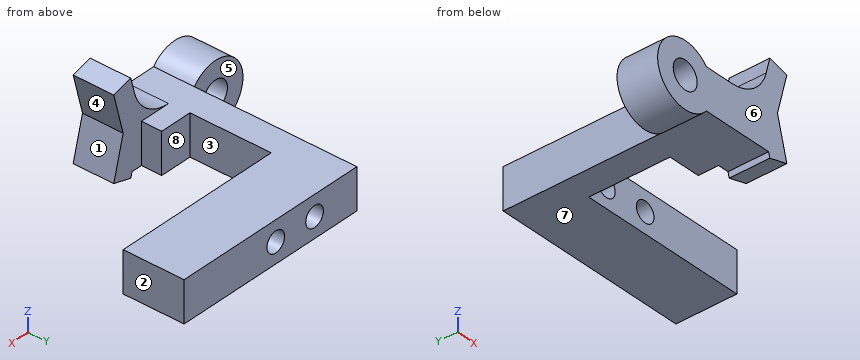
```python
from build123d import *

# Parameters (mm, degrees)
BOSS_EXTRUDE1_DEPTH = 5
BOSS_EXTRUDE2_DEPTH = 10
FILLET1_R           = 10
SKETCH3_W           = 8
SKETCH3_H           = 20
CUT_EXTRUDE1_DEPTH  = 74.171272574
SKETCH4_R           = 2.5
CUT_EXTRUDE2_DEPTH  = 63.379394923
SKETCH5_R           = 3.4
BOSS_EXTRUDE4_DEPTH = 10


with BuildPart() as part:
    # Sketch1 → Boss-Extrude1 (new, symmetric)
    with BuildSketch(Plane.XY):
        Polygon((49, 0), (0, 0), (0, -50), (15, -50), (15, -15), (49, -15), align=None)
    extrude(amount=BOSS_EXTRUDE1_DEPTH, both=True)

    # Sketch2 → Boss-Extrude2 (add)
    with BuildSketch(Plane.XZ.offset(50)):
        Polygon((22.832157544, -5), (18, -6.284621916), (15, 5), (18, 16.284621916), (22.832157544, 15), (20.173672375, 5), align=None)
        Polygon((15, -5), (17.658485169, -5), (15, 5), align=None)
        Polygon((18, 16.284621916), (15, 5), (20.173672375, 5), (22.832157544, 15), align=None)
    extrude(amount=-BOSS_EXTRUDE2_DEPTH)

    # Fillet1
    fillet1_edges = [part.edges().sort_by_distance(p)[0] for p in [
        (15, -45, 5),
    ]]
    fillet(fillet1_edges, radius=FILLET1_R)

    # Sketch3 → Cut-Extrude1 (cut, through all)
    with BuildSketch(Plane(origin=(0, 0, -5), x_dir=(-1, 0, 0), z_dir=(0, 0, -1))):
        with Locations((-11, -25)):
            Rectangle(SKETCH3_W, SKETCH3_H)
    extrude(amount=-CUT_EXTRUDE1_DEPTH, mode=Mode.SUBTRACT)

    # Sketch4 → Cut-Extrude2 (cut, through all)
    with BuildSketch(Plane.XZ.offset(15)):
        with Locations(Location((23, 0, 0), (0, 0, 270))):
            Circle(SKETCH4_R)
        with Locations(Location((12, 0, 0), (0, 0, 270))):
            Circle(SKETCH4_R)
    extrude(amount=-CUT_EXTRUDE2_DEPTH, mode=Mode.SUBTRACT)

    # Sketch5 → Boss-Extrude4 (add)
    with BuildSketch(Plane.XZ.offset(50)):
        with BuildLine():
            Line((0, 5), (0, -5))
            ThreePointArc((0, -5), (-13.810249676, 0), (0, 5))
        make_face()
        with Locations(Location((-6, 0, 0), (0, 0, 270))):
            Circle(SKETCH5_R, mode=Mode.SUBTRACT)
    extrude(amount=-BOSS_EXTRUDE4_DEPTH)


solid = part.part
```
Part model, mm, in its own coordinate system. Face numbers are marked on the shaded views. A direction names the side the tool comes from. Round coordinates to 2 decimals unless told otherwise and drop trailing zeros. Loops run counter-clockwise (first coordinate to the right, second up) from the corner with the lowest first, then second, coordinate; pieces in that order, holes last. Notation, with made-up numbers: (41, -3.5) -> (96, -3.5) arc R5 ccw to (96, 4.5) -> close; hole circle Ø4 at (67, -19.5). An arc over 180 degrees is marked (long way). Use one line per item in the form item = value. Start each with the question number.
Item 1: Drop flat-ended pins along their axis: pin 1 Ø3 at (x, z) = (36, -1) entering from -Y; pin 2 Ø12 at (x, z) = (24.5, 6.5) entering from +Y; pin 3 Ø8 at (x, z) = (-6, 0) entering from +Y; pin 4 Ø14.5 at (x, y) = (29, -28) entering from -Z. Give the stop position or say it passes through.
Item 2: Drill centre lines: line 1 along X through (y, z) = (-9, 0); line 2 along Y through (x, z) = (7.5, 0.25); line 3 along Y through (x, z) = (-2.5, 1.5). Where is each one in solid material? Low to high.
Item 3: Band-saw the part on A-A (x = -6). List the corners of the cut face in (y, z), plus the area to 3 significant figures.
Item 4: Band-saw the part on B-B (y = -46). List the corners of the cut face in (x, z).
Item 5: Band-saw the part on D-D (z = 0). List the corners of the cut face in (x, y), plus the area to 3 significant figures.
Item 6: Tool access for the marked faces 1, 2, 3, 4 and 5: list every direction of +Z, -Z, +X, -X, +Y, -Y with a clear straight run to the whole face (end or side of a thin tool).
Item 7: Two-plate mould, pull along Y, no slides. Class the marked faces 6, 7 and 8: released by +Y, released by -Y, zero draft, split by the parting line, or undercut.
Item 8: Band-saw the part on C-C (y = -8). List the corners of the cut face in (x, z).
Data:
q1.pin_1 = -15
q1.pin_2 = 0
q1.pin_3 = -40
q1.pin_4 = through
q2.line_1 = 0 to 9.5, 14.5 to 20.5, 25.5 to 49
q2.line_2 = -50 to -35, -15 to 0
q2.line_3 = -50 to -40
q3.outline = (-50, -7.81) -> (-40, -7.81) -> (-40, -3.4) -> (-50, -3.4) -> close; (-50, 3.4) -> (-40, 3.4) -> (-40, 7.81) -> (-50, 7.81) -> close
q3.area = 88.2 mm^2
q4.outline = (0, -5) -> (17.66, -5) -> (18, -6.28) -> (22.83, -5) -> (20.17, 5) -> (22.83, 15) -> (18, 16.28) -> (16.98, 12.43) arc R10 cw to (7.31, 5) -> (0, 5) arc R7.81 ccw (long way) to start; hole circle Ø6.8 at (-6, 0)
q5.outline = (-13.81, -50) -> (-9.4, -50) -> (-9.4, -40) -> (-13.81, -40) -> close; (-2.6, -50) -> (21.5, -50) -> (21.5, -40) -> (15, -40) -> (15, -35) -> (7, -35) -> (7, -15) -> (9.5, -15) -> (9.5, 0) -> (0, 0) -> (0, -40) -> (-2.6, -40) -> close; (14.5, -15) -> (20.5, -15) -> (20.5, 0) -> (14.5, 0) -> close; (25.5, -15) -> (49, -15) -> (49, 0) -> (25.5, 0) -> close
q5.area = 1,090 mm^2
q6.face_1 = +X, -Y
q6.face_2 = +Z, -Z, +X, +Y, -Y
q6.face_3 = +Z, -Z, +X
q6.face_4 = +X, +Y, -Y
q6.face_5 = +Z, -Z, -X, +Y
q7.face_6 = released by -Y
q7.face_7 = zero draft
q7.face_8 = undercut
q8.outline = (0, -5) -> (49, -5) -> (49, 5) -> (0, 5) -> close; hole circle Ø5 at (12, 0); hole circle Ø5 at (23, 0)
